Verification items for this drawing (mm, ordinates from the low corner). A direction names the side the tool comes from. Round coordinates to 2 decimals unless told otherwise and drop trailing zeros. Loops run counter-clockwise (first coordinate to the right, second up) from the corner with the lowest first, then second, coordinate; pieces in that order, holes last. Notation, with made-up numbers: (58, 13.25) -> (82, 13.25) arc R13 cw to (82, 31.25) -> close; hole circle Ø3 at (25.25, 30.5). An arc over 180 degrees is marked (long way). Use a Markdown table: item, result. Add a question column.
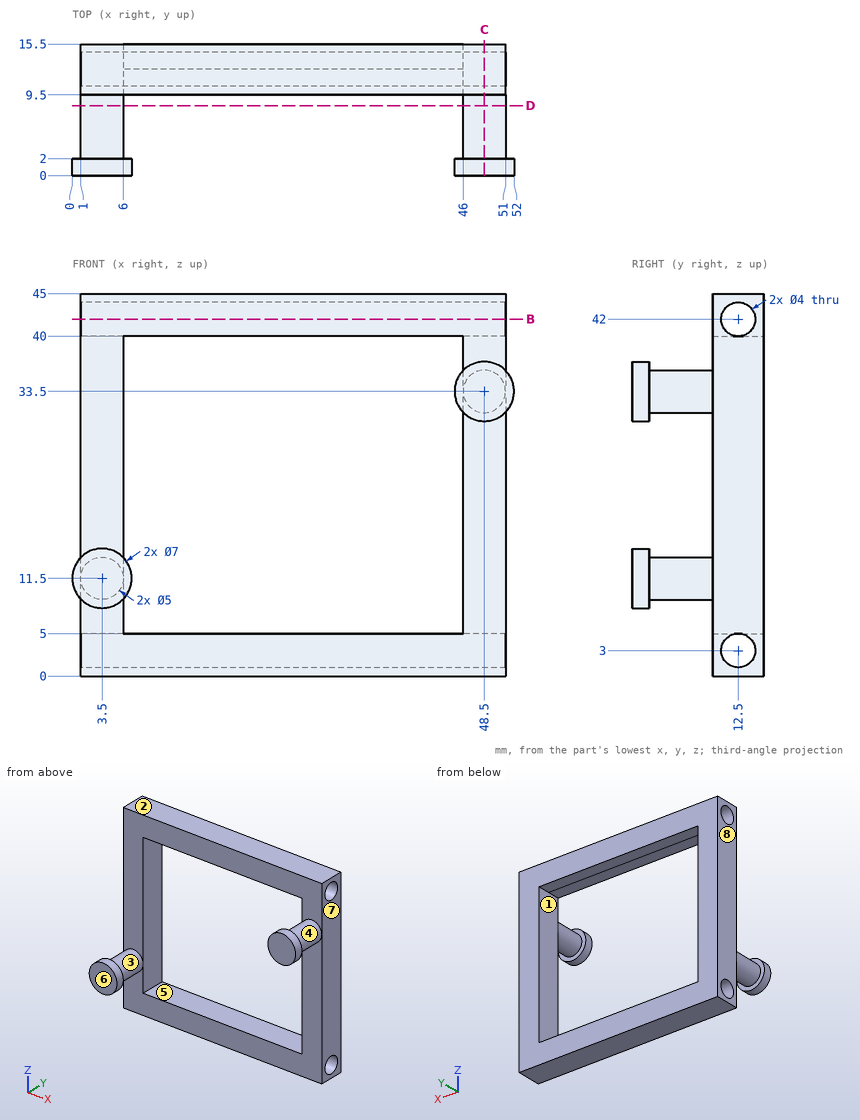
1) Thickness scan on line 1 (Z direction, x = 21.5, y = 9.75); line 2 (Y direction, x = 19, z = 42); line 3 (X direction, y = 11.75, z = 12). Record the ranges inside material, lowest first.
2) Release check for a two-part mould opening along Z. For the marked faces 1, 2 and 3 record: released by +Z, released by -Z, zero draft, split by the parting line, or undercut.
3) Access from +Z, -Z, +X, -X, +Y, -Y to the whole of each face (thin tool, end or side, straight path). Record for the marked faces 4, 5, 6, 7 and 8.
4) Sectioned sample at B-B on z = 42. Enter the section's corners in (x, y), then the cut area to 3 significant figures.
5) Sectioned sample at C-C on x = 48.5. Enter the section's corners in (y, z), then the cut area to 3 significant figures.
6) Sectioned sample at D-D on y = 8.25. Enter the section's corners in (x, z), then the cut area to 3 significant figures.
7) Go/stop test with flat-tipped pins: pin 1 (6.5 mm diameter, centred on y = 12, z = 14.5, fed in from +X); pin 2 (1.5 mm diameter, centred on x = 31, y = 14.5, fed in from -Z); pin 3 (4.5 mm diameter, centred on y = 12.5, z = 42, fed in from -X); pin 4 (17 mm diameter, centred on x = 25, z = 13, fed in from -Y). Record where each tip stops, or that it passes through.
Geometry results:
| question | item | result |
|---|---|---|
| 1 | line 1 | 0 to 5, 40 to 45 |
| 1 | line 2 | 9.5 to 10.5, 14.5 to 15.5 |
| 1 | line 3 | 1 to 6, 46 to 51 |
| 2 | face 1 | undercut |
| 2 | face 2 | released by +Z |
| 2 | face 3 | split by the parting line |
| 3 | face 4 | none |
| 3 | face 5 | +Y, -Y |
| 3 | face 6 | +Z, -Z, +X, -X, -Y |
| 3 | face 7 | +Z, -Z, +X, +Y |
| 3 | face 8 | +Z, -Z, -X, +Y |
| 4 | outline | (1, 9.5) -> (51, 9.5) -> (51, 10.5) -> (1, 10.5) -> close; (1, 14.5) -> (51, 14.5) -> (51, 15.5) -> (1, 15.5) -> close |
| 4 | area | 100 mm^2 |
| 5 | outline | (0, 30) -> (2, 30) -> (2, 31) -> (9.5, 31) -> (9.5, 0) -> (15.5, 0) -> (15.5, 45) -> (9.5, 45) -> (9.5, 36) -> (2, 36) -> (2, 37) -> (0, 37) -> close; hole circle Ø4 at (12.5, 3); hole circle Ø4 at (12.5, 42) |
| 5 | area | 296 mm^2 |
| 6 | outline | circle Ø5 at (3.5, 11.5); circle Ø5 at (48.5, 33.5) |
| 6 | area | 39.3 mm^2 |
| 7 | pin 1 | x = 51 |
| 7 | pin 2 | z = 0 |
| 7 | pin 3 | x = 1 |
| 7 | pin 4 | y = 9.5 |
